from build123d import *

# Parameters (mm, degrees)
SKETCH1_W           = 172
SKETCH1_H           = 4
BOSS_EXTRUDE1_DEPTH = 50
CUT_EXTRUDE1_DEPTH  = 50
SKETCH3_W           = 35
SKETCH3_H           = 73
BOSS_EXTRUDE2_DEPTH = 3
SKETCH4_W           = 2.8
SKETCH4_H           = 15
SKETCH4_W_2         = 6
BOSS_EXTRUDE3_DEPTH = 20
FILLET1_R           = 7
SKETCH5_R           = 2.75
CUT_EXTRUDE2_DEPTH  = 30
SKETCH6_W           = 5.6
SKETCH6_H           = 73
SKETCH6_W_2         = 7.6
CUT_EXTRUDE3_DEPTH  = 20
SKETCH7_W           = 6
SKETCH7_H           = 58
BOSS_EXTRUDE4_DEPTH = 10
CHAMFER1_SIZE       = 10
CHAMFER2_SIZE       = 15
FILLET2_R           = 5
SKETCH8_W           = 172
SKETCH8_H           = 4
BOSS_EXTRUDE5_DEPTH = 2
CHAMFER3_SIZE       = 3
CHAMFER4_SIZE       = 5


with BuildPart() as part:
    # Sketch1 → Boss-Extrude1 (new body)
    with BuildSketch(Plane.XY):
        Rectangle(SKETCH1_W, SKETCH1_H)
    extrude(amount=BOSS_EXTRUDE1_DEPTH)

    # Sketch2 → Cut-Extrude1 (cut)
    with BuildSketch(Plane(origin=(0, 2, 0), x_dir=(1, 0, 0), z_dir=(0, 1, 0))):
        with BuildLine():
            Line((-76.5, -10.45), (-74.65, -10.45))
            ThreePointArc((-74.65, -10.45), (-72.8, -12.3), (-74.65, -14.15))
            Line((-74.65, -14.15), (-76.5, -14.15))
            ThreePointArc((-76.5, -14.15), (-78.35, -12.3), (-76.5, -10.45))
        make_face()
        with BuildLine():
            Line((74.65, -10.45), (76.5, -10.45))
            ThreePointArc((76.5, -10.45), (78.35, -12.3), (76.5, -14.15))
            Line((76.5, -14.15), (74.65, -14.15))
            ThreePointArc((74.65, -14.15), (72.8, -12.3), (74.65, -10.45))
        make_face()
        with BuildLine():
            Line((-76.5, -35.85), (-74.65, -35.85))
            ThreePointArc((-74.65, -35.85), (-72.8, -37.7), (-74.65, -39.55))
            Line((-74.65, -39.55), (-76.5, -39.55))
            ThreePointArc((-76.5, -39.55), (-78.35, -37.7), (-76.5, -35.85))
        make_face()
        with BuildLine():
            Line((74.65, -35.85), (76.5, -35.85))
            ThreePointArc((76.5, -35.85), (78.35, -37.7), (76.5, -39.55))
            Line((76.5, -39.55), (74.65, -39.55))
            ThreePointArc((74.65, -39.55), (72.8, -37.7), (74.65, -35.85))
        make_face()
    extrude(amount=-CUT_EXTRUDE1_DEPTH, mode=Mode.SUBTRACT)

    # Sketch3 → Boss-Extrude2 (add)
    with BuildSketch(Plane.XY.offset(50)):
        with Locations((43.1, -38.5)):
            Rectangle(SKETCH3_W, SKETCH3_H)
    extrude(amount=-BOSS_EXTRUDE2_DEPTH)

    # Sketch4 → Boss-Extrude3 (add)
    with BuildSketch(Plane(origin=(0, 0, 47), x_dir=(-1, 0, 0), z_dir=(0, 0, -1))):
        with Locations((-44.1, -67.5)):
            Rectangle(SKETCH4_W, SKETCH4_H)
        with Locations((-36.2, -67.5)):
            Rectangle(SKETCH4_W_2, SKETCH4_H)
        with Locations((-52, -67.5)):
            Rectangle(SKETCH4_W_2, SKETCH4_H)
    extrude(amount=BOSS_EXTRUDE3_DEPTH)

    # Fillet1
    fillet1_edges = [part.edges().sort_by_distance(p)[0] for p in [
        (44.1, -75, 27),
        (44.1, -60, 27),
        (36.2, -75, 27),
        (36.2, -60, 27),
        (52, -60, 27),
        (52, -75, 27),
    ]]
    fillet(fillet1_edges, radius=FILLET1_R)

    # Sketch5 → Cut-Extrude2 (cut)
    with BuildSketch(Plane(origin=(55, 0, 0), x_dir=(0, 0, -1), z_dir=(1, 0, 0))):
        with Locations((-34, -67)):
            Circle(SKETCH5_R)
    extrude(amount=-CUT_EXTRUDE2_DEPTH, mode=Mode.SUBTRACT)

    # Sketch6 → Cut-Extrude3 (cut)
    with BuildSketch(Plane(origin=(0, 0, 47), x_dir=(-1, 0, 0), z_dir=(0, 0, -1))):
        with Locations((-57.8, -38.5)):
            Rectangle(SKETCH6_W, SKETCH6_H)
        with Locations((-29.4, -38.5)):
            Rectangle(SKETCH6_W_2, SKETCH6_H)
    extrude(amount=-CUT_EXTRUDE3_DEPTH, mode=Mode.SUBTRACT)

    # Sketch7 → Boss-Extrude4 (add)
    with BuildSketch(Plane(origin=(0, 0, 47), x_dir=(-1, 0, 0), z_dir=(0, 0, -1))):
        with Locations((-52, -31)):
            Rectangle(SKETCH7_W, SKETCH7_H)
        with Locations((-36.2, -31)):
            Rectangle(SKETCH7_W, SKETCH7_H)
    extrude(amount=BOSS_EXTRUDE4_DEPTH)

    # Chamfer1
    chamfer1_edges = [part.edges().sort_by_distance(p)[0] for p in [
        (44.1, -60, 47),
    ]]
    chamfer(chamfer1_edges, length=CHAMFER1_SIZE)

    # Chamfer2
    chamfer2_edges = [part.edges().sort_by_distance(p)[0] for p in [
        (52, -2, 37),
        (36.2, -2, 37),
    ]]
    chamfer(chamfer2_edges, length=CHAMFER2_SIZE)

    # Fillet2
    fillet2_edges = [part.edges().sort_by_distance(p)[0] for p in [
        (55, -2, 36),
        (33.2, -2, 36),
    ]]
    fillet(fillet2_edges, radius=FILLET2_R)

    # Sketch8 → Boss-Extrude5 (add)
    with BuildSketch(Plane(origin=(0, 2, 0), x_dir=(1, 0, 0), z_dir=(0, 1, 0))):
        with Locations((0, -2)):
            Rectangle(SKETCH8_W, SKETCH8_H)
        with Locations((0, -48)):
            Rectangle(SKETCH8_W, SKETCH8_H)
    extrude(amount=BOSS_EXTRUDE5_DEPTH)

    # Chamfer3
    # the kernel refuses this chamfer: 3 mm, written as the material it adds along each edge
    with BuildSketch(Plane(origin=(-86, 2, 46), x_dir=(0, -0.027495876610586334, -0.9996219169112968), z_dir=(1, 0, 0))) as chamfer3_piece_1_section:
        Polygon((CHAMFER3_SIZE * 0.999621916911, CHAMFER3_SIZE * 0.0274958766106), (-CHAMFER3_SIZE * 0.0274958766106, CHAMFER3_SIZE * 0.999621916911), (0, 0), align=None)
    chamfer3_piece_1 = extrude(amount=172, mode=Mode.PRIVATE)
    chamfer3_piece_1 = split(chamfer3_piece_1, bisect_by=Plane(origin=(0, 4, 44.907908995), z_dir=(0, -1, 0)), keep=Keep.TOP, mode=Mode.PRIVATE)
    add(chamfer3_piece_1)
    with BuildSketch(Plane(origin=(86, 2, 4), x_dir=(0, -0.02749587661058634, 0.9996219169112968), z_dir=(-1, 0, 0))) as chamfer3_piece_2_section:
        Polygon((CHAMFER3_SIZE * 0.999621916911, CHAMFER3_SIZE * 0.0274958766106), (-CHAMFER3_SIZE * 0.0274958766106, CHAMFER3_SIZE * 0.999621916911), (0, 0), align=None)
    chamfer3_piece_2 = extrude(amount=172, mode=Mode.PRIVATE)
    chamfer3_piece_2 = split(chamfer3_piece_2, bisect_by=Plane(origin=(0, 4, 5.092091005), z_dir=(0, -1, 0)), keep=Keep.TOP, mode=Mode.PRIVATE)
    add(chamfer3_piece_2)

    # Chamfer4
    chamfer4_edges = [part.edges().sort_by_distance(p)[0] for p in [
        (-86, 1, 0),
        (-86, 1, 50),
        (86, 1, 50),
        (86, 1, 0),
    ]]
    chamfer(chamfer4_edges, length=CHAMFER4_SIZE)


solid = part.part
CAD build for the part. Positions are in the model's coordinates, mm. A direction names the side the tool comes from. Give positions to 0.01 mm unless a question says otherwise; leave off trailing zeros. Write each loop counter-clockwise with the first axis right and the second up, starting at its lowest first coordinate (ties: lowest second). Pieces come first, ordered by that corner, then holes. Notation, with made-up numbers: M 29,18.5 L 48,18.5 A12 cw 48,37.5 Z; hole C -38.75,30 d6. An arc over 180 degrees is marked long. Put each result on its own line as item: value. Start each with the question number.
(1) Band-saw the part on D-D, the plane x = -67. Write the cut outline in (y, z), and give its area (3 significant figures).
(2) Band-saw the part on B-B, the plane y = -30. Write the cut outline in (x, z), and give its area (3 significant figures).
(3) Mould opens along X. For faces 4 (the face through (52, -60, 36)), 5 (the face through (39.2, -39, 40)), 6 (the face through (-86, 0, 25)) say: +X half, -X half, draft (parallel to the pull), parting line (faces both ways), or undercut.
(4) Probe L1, parallel to X at y = -56, z = 44.5; L2, parallel to X at y = -19.5, z = 43; L3, parallel to Y at x = 35.95, z = 34. List the from-to ranges inside material, lowest first.
(5) Which spindle directions (+Z, -Z, +X, -X, +Y, -Y) get a long thin tool onto all of the face, cutting with end or side? Do faces 1 (the face through (-1, 2, 25)), 2 (the face through (52, -62, 29.1)), 3 (the face through (-78.35, 0.03, 12.34)). Say none if no direction does.
(6) Band-saw the part on C-C, the plane z = 29. Write the cut outline in (x, y), and give its area (3 significant figures).
(7) Flat gauge pins, fed straight in: pin 1 Ø10 at (y, z) = (-55, 44) entering from +X; pin 2 Ø5 at (x, y) = (52, -44) entering from -Z; pin 3 Ø3.5 at (x, z) = (52, 35) entering from +Y. Where does each tip first touch, or does it go through?
(8) Band-saw the part on A-A, the plane z = 12.3. Write the cut outline in (x, y).
Response values:
1. outline: M -2,0 L 4,0 L 4,5 L 2,7 L 2,43 L 4,45 L 4,50 L -2,50 Z
1. area: 224 mm2
2. outline: M 33.2,37 L 39.2,37 L 39.2,47 L 49,47 L 49,37 L 55,37 L 55,50 L 33.2,50 Z
2. area: 185 mm2
3. face 4: draft
3. face 5: undercut
3. face 6: -X half
4. L1: x = 33.2 to 39.2, 42.7 to 45.5, 49 to 55
4. L2: x = 33.2 to 39.2, 49 to 55
4. L3: y = -75 to -69.75, -64.25 to -60, -14 to 2
5. face 1: +X, -X, +Y
5. face 2: -Z, +X, -X
5. face 3: +Y, -Y
6. outline: M -86,-2 L 28.2,-2 A5 cw 33.2,-7 L 33.2,-9 L 39.2,-9 L 39.2,-2 L 49,-2 L 49,-9 L 55,-9 L 55,-7 A5 cw 60,-2 L 86,-2 L 86,2 L -86,2 Z; M 33.2,-72.9 L 39.2,-72.9 L 39.2,-62.1 L 33.2,-62.1 Z; M 42.7,-72.9 L 45.5,-72.9 L 45.5,-62.1 L 42.7,-62.1 Z; M 49,-72.9 L 55,-72.9 L 55,-62.1 L 49,-62.1 Z
6. area: 943 mm2
7. pin 1: stops at x = 55
7. pin 2: stops at z = 37
7. pin 3: stops at y = 2
8. outline: M -86,-2 L -78.35,-2 L -78.35,2 L -86,2 Z; M -72.8,-2 L 72.8,-2 L 72.8,2 L -72.8,2 Z; M 78.35,-2 L 86,-2 L 86,2 L 78.35,2 Z
